```python
from build123d import *

# Parameters (mm, degrees)
SKETCH1_W           = 30
SKETCH1_H           = 20
BOSS_EXTRUDE1_DEPTH = 11
SKETCH2_W           = 30
SKETCH2_H           = 6.5
CUT_EXTRUDE1_DEPTH  = 17.5
FILLET1_R           = 1


with BuildPart() as part:
    # Sketch1 → Boss-Extrude1 (new body)
    with BuildSketch(Plane(origin=(0, 0, 0), x_dir=(1, 0, 0), z_dir=(0, 1, 0))):
        Rectangle(SKETCH1_W, SKETCH1_H)
    extrude(amount=BOSS_EXTRUDE1_DEPTH)

    # Sketch2 → Cut-Extrude1 (cut)
    with BuildSketch(Plane.XY.offset(10)):
        with Locations((0, 5.5)):
            Rectangle(SKETCH2_W, SKETCH2_H)
    extrude(amount=-CUT_EXTRUDE1_DEPTH, mode=Mode.SUBTRACT)

    # Fillet1
    fillet1_edges = [part.edges().sort_by_distance(p)[0] for p in [
        (-15, 11, 0),
        (0, 11, 10),
        (15, 1.125, 10),
        (-15, 1.125, 10),
        (-15, 8.75, 1.25),
        (15, 5.5, -7.5),
        (15, 8.75, 1.25),
        (15, 2.25, 1.25),
        (-15, 5.5, -7.5),
        (-15, 2.25, 1.25),
        (0, 8.75, 10),
        (0, 2.25, 10),
        (15, 11, 0),
        (0, 0, 10),
        (-15, 0, 0),
        (0, 0, -10),
        (15, 0, 0),
        (0, 11, -10),
        (15, 9.875, 10),
        (-15, 9.875, 10),
        (-15, 5.5, -10),
        (15, 5.5, -10),
    ]]
    fillet(fillet1_edges, radius=FILLET1_R)


solid = part.part
```
Read the model definition and answer for the solid it produces. Units are mm, in the model's axes. A direction names the side the tool comes from. Coordinates: 2 decimals unless noted, no trailing zeros. Loops run counter-clockwise (first coordinate to the right, second up) from the corner with the lowest first, then second, coordinate; pieces in that order, holes last. Notation, with made-up numbers: (-0.75, 60) - (51.25, 60) arc R29 cw to (51.25, 83) - close; hole circle Ø8 at (87.25, 0.25). An arc over 180 degrees is marked (long way). Answer in a Markdown table with one row per item.
1. Find section C-C, the plane y = 6. Write down the section's boundary in (x, z).
Conclusion:
| item | result |
|---|---|
| outline | (-15, -9) arc R1 ccw to (-14, -10) - (14, -10) arc R1 ccw to (15, -9) - (15, -8.5) arc R1 ccw to (14, -7.5) - (-14, -7.5) arc R1 ccw to (-15, -8.5) - close |
2. Find section B-B, the plane x = 10. Write down the section's boundary in (y, z).
Conclusion:
| item | result |
|---|---|
| outline | (0, -9) arc R1 ccw to (1, -10) - (10, -10) arc R1 ccw to (11, -9) - (11, 9) arc R1 ccw to (10, 10) - (9.75, 10) arc R1 ccw to (8.75, 9) - (8.75, -7.5) - (2.25, -7.5) - (2.25, 9) arc R1 ccw to (1.25, 10) - (1, 10) arc R1 ccw to (0, 9) - close |
3. Find section A-A, the plane z = 7.25. Write down the section's boundary in (x, y), then the cut area to 3 significant figures.
Conclusion:
| item | result |
|---|---|
| outline | (-15, 1) arc R1 ccw to (-14, 0) - (14, 0) arc R1 ccw to (15, 1) - (15, 1.25) arc R1 ccw to (14, 2.25) - (-14, 2.25) arc R1 ccw to (-15, 1.25) - close; (-15, 9.75) arc R1 ccw to (-14, 8.75) - (14, 8.75) arc R1 ccw to (15, 9.75) - (15, 10) arc R1 ccw to (14, 11) - (-14, 11) arc R1 ccw to (-15, 10) - close |
| area | 133 mm² |
4. Given pin 1 (3 mm diameter, centred on x = -2.5, y = 3, fed in from +Z); pin 2 (3 mm diameter, centred on x = -5, y = 7, fed in from +Z); pin 3 (1 mm diameter, centred on y = 9, z = -7, fed in from -X), each flat-ended and moving along its own axis, determine where each tip first touches the part or whether it passes through.
Conclusion:
| item | result |
|---|---|
| pin 1 | stops at z = 9.97 |
| pin 2 | stops at z = -7.5 |
| pin 3 | stops at x = -14.97 |
5. Straight lines are drawn through the part: line 1 (Y direction, x = 0.25, z = -4.75); line 2 (Z direction, x = 10.25, y = 8); line 3 (X direction, y = 10.75, z = -2.75). For each, find the intervals that lie inside material, in ascending order.
Conclusion:
| item | result |
|---|---|
| line 1 | y = 0 to 2.25, 8.75 to 11 |
| line 2 | z = -10 to -7.5 |
| line 3 | x = -14.66 to 14.66 |
6. Which of the six approach directions +Z, -Z, +X, -X, +Y, -Y give full straight-line access (tool end or side, diameter ignored) to faces 1 (the face through (14.699, 5.56, -7.785)), 2 (the face through (0, 2.25, 1)), 3 (the face through (-14.715, 1.949, 0.127))?
Conclusion:
| item | result |
|---|---|
| face 1 | +Z, +X |
| face 2 | +Z, +X, -X |
| face 3 | +Z, -X |
7. Determine the mould class of faces 4 (the face through (0.196, 10.715, 9.699)), 5 (the face through (0, 8.75, 1)), 6 (the face through (0, 5, -10)), 7 (the face through (0, 0, 0)) for opening direction Y: +Y half, -Y half, draft (parallel to the pull), parting line (faces both ways), or undercut.
Conclusion:
| item | result |
|---|---|
| face 4 | +Y half |
| face 5 | undercut |
| face 6 | draft |
| face 7 | -Y half |
